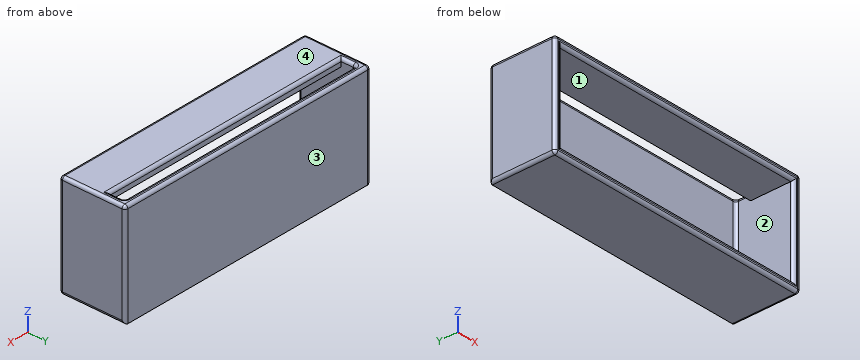
```python
from build123d import *

# Parameters (mm, degrees)
F0_W     = 914.4
F0_H     = 349.25
F1_DEPTH = 222.25
F2_T     = -25.4
F3_W     = 863.6
F3_H     = 50.8
F4_DEPTH = 25.4
F5_R     = 10.16


with BuildPart() as f1:
    # F0 (on Front) → F1 (new body)
    with BuildSketch(Plane.XZ):
        Rectangle(F0_W, F0_H)
    extrude(amount=F1_DEPTH)

    # F2
    f2_openings = [f1.faces().sort_by_distance(p)[0] for p in [
        (0, -222.25, 0),
    ]]
    offset(amount=F2_T, openings=f2_openings)

    # F3 (on face) → F4 (cut)
    with BuildSketch(Plane.XY.offset(174.625)):
        with Locations((0, -50.8)):
            Rectangle(F3_W, F3_H)
    extrude(amount=-F4_DEPTH, mode=Mode.SUBTRACT)

    # F5
    f5_edges = [f1.edges().sort_by_distance(p)[0] for p in [
        (457.2, -111.125, 174.625),
        (0, 0, 174.625),
        (457.2, 0, 0),
        (457.2, -111.125, -174.625),
        (457.2, -222.25, 0),
        (431.8, -25.4, 12.7),
        (0, -25.4, -149.225),
        (-431.8, -25.4, 12.7),
        (0, -25.4, 174.625),
        (0, -222.25, 174.625),
        (-457.2, -222.25, 0),
        (0, -222.25, -174.625),
        (431.8, -222.25, 0),
        (0, -222.25, -149.225),
        (-431.8, -222.25, 0),
        (0, -222.25, 149.225),
        (-457.2, 0, 0),
        (-457.2, -111.125, 174.625),
        (-457.2, -111.125, -174.625),
        (0, -76.2, 174.625),
        (-431.8, -50.8, 174.625),
        (431.8, -50.8, 174.625),
    ]]
    fillet(f5_edges, radius=F5_R)


solid = f1.part
```
Design review of the part built by this model. Coordinates are the model's own, in mm. Face numbers are marked on the shaded views. Coordinates: 2 decimals unless noted, no trailing zeros. Loops run counter-clockwise (first coordinate to the right, second up) from the corner with the lowest first, then second, coordinate; pieces in that order, holes last. Notation, with made-up numbers: (16, 5) -> (48, 5) arc R14 ccw to (48, 9) -> close; hole circle Ø8 at (-33, 88.5). An arc over 180 degrees is marked (long way). Answer as a JSON object with one key per item and string values.
Q1. Take a section at B-B on y = -157.5. Give the boundary of the cut face in (x, z) (3 decimals).
Answer block:
{"outline": "(-457.2, -164.465) arc R10.16 ccw to (-447.04, -174.625) -> (447.04, -174.625) arc R10.16 ccw to (457.2, -164.465) -> (457.2, 164.465) arc R10.16 ccw to (447.04, 174.625) -> (-447.04, 174.625) arc R10.16 ccw to (-457.2, 164.465) -> close; hole (-431.8, -149.225) -> (431.8, -149.225) -> (431.8, 149.225) -> (-431.8, 149.225) -> close"}
Q2. Take a section at C-C on z = -17. Give the boundary of the cut face in (x, y), plus the area to 3 significant figures.
Answer block:
{"outline": "(-457.2, -212.09) arc R10.16 ccw to (-447.04, -222.25) -> (-441.96, -222.25) arc R10.16 ccw to (-431.8, -212.09) -> (-431.8, -35.56) arc R10.16 cw to (-421.64, -25.4) -> (421.64, -25.4) arc R10.16 cw to (431.8, -35.56) -> (431.8, -212.09) arc R10.16 ccw to (441.96, -222.25) -> (447.04, -222.25) arc R10.16 ccw to (457.2, -212.09) -> (457.2, -10.16) arc R10.16 ccw to (447.04, 0) -> (-447.04, 0) arc R10.16 ccw to (-457.2, -10.16) -> close", "area": "33,100 mm^2"}
Q3. To check wall thickness, follow L1, parallel to X at y = -65, z = 35; L2, parallel to Z at x = -93, y = -121 (3 decimals); L3, parallel to Y at x = -87, z = -36.5. State the ranges of each line that lie inside material, in increasing order.
Answer block:
{"L1": "x = -457.2 to -431.8, 431.8 to 457.2", "L2": "z = -174.625 to -149.225, 149.225 to 174.625", "L3": "y = -25.4 to 0"}
Q4. Take a section at A-A on x = 150.5. Give the boundary of the cut face in (y, z) (3 decimals), plus the area to 3 significant figures.
Answer block:
{"outline": "(-222.25, -164.465) arc R10.16 ccw to (-212.09, -174.625) -> (0, -174.625) -> (0, 164.465) arc R10.16 ccw to (-10.16, 174.625) -> (-15.24, 174.625) arc R10.16 ccw to (-25.4, 164.465) -> (-25.4, -139.065) arc R10.16 cw to (-35.56, -149.225) -> (-212.09, -149.225) arc R10.16 ccw to (-222.25, -159.385) -> close; (-222.25, 159.385) arc R10.16 ccw to (-212.09, 149.225) -> (-76.2, 149.225) -> (-76.2, 164.465) arc R10.16 ccw to (-86.36, 174.625) -> (-212.09, 174.625) arc R10.16 ccw to (-222.25, 164.465) -> close", "area": "17,400 mm^2"}
Q5. Clearance check with a flat-ended pin moving along its axis: pin 1 Ø10 at (x, z) = (-8.5, 104.5) entering from -Y. State where the tip first meets the part, or that it passes through.
Answer block:
{"pin 1": "stops at y = -25.4"}
Q6. The part is to be moulded in two halves that separate along Z. For the marked faces 1, 2, 3 and 4, say which applies: +Z half, -Z half, draft (parallel to the pull), parting line (faces both ways), or undercut.
Answer block:
{"face 1": "undercut", "face 2": "undercut", "face 3": "draft", "face 4": "+Z half"}
